Can you work these out from the model? Positions are in its coordinate system, mm. Coordinates: 2 decimals unless noted, no trailing zeros. Order: outer loops, then holes, each group sorted by start corner. A loop starts at its lowest first (then second) coordinate and runs counter-clockwise, first axis right, second up. Notation, with made-up numbers: (77.25, 86) -> (92.25, 86) arc R18 cw to (92.25, 112) -> close; hole circle Ø1 at (-32.75, 25.5). An arc over 180 degrees is marked (long way). Answer in a Markdown table with one row per item. Add a question column.
1. Imagine slicing it at B-B on x = 2.54. Write out the boundary of the cut face in (y, z), plus the area to 3 significant figures.
2. Will this pin go through, and if not, where does the flat tip stop? pin 1 (2.5 mm diameter, centred on x = 2.54, z = -3.048, fed in from +Y).
3. If I drill on line 1 along X through (y, z) = (0.45, -10.75); line 2 along X through (y, z) = (0.75, -12); line 3 along Z through (x, y) = (3.5, 0.25), over which ranges is the centre line in solid material (lowest first)? Write a range as [from, to].
4. Imagine slicing it at D-D on z = -6.25. Write out the boundary of the cut face in (x, y), plus the area to 3 significant figures.
5. We'd pull the mould along Z, two halves only. Please class faces 1 (the face through (13, 1, 0)), 2 (the face through (12.878, 1.252, -7.536)), 3 (the face through (2.998, 1.252, -9.214)): pulls with the +Z half, pulls with the -Z half, needs draft (parallel to the pull), parting line crosses it, or undercut.
6. Imagine slicing it at C-C on z = -11.75. Write out the boundary of the cut face in (x, y), plus the area to 3 significant figures.
7. Imagine slicing it at A-A on y = 2. Write out the boundary of the cut face in (x, z), plus the area to 3 significant figures.
from build123d import *

# Parameters (mm, degrees)
SKETCH1_R           = 1.524
BOSS_EXTRUDE1_DEPTH = 2.54


with BuildPart() as part:
    # Sketch1 → Boss-Extrude1 (new body)
    with BuildSketch(Plane(origin=(0, 0, 0), x_dir=(1, 0, 0), z_dir=(0, 1, 0))):
        Polygon((0, 0), (25.4, 0), (0, 15.285917978), align=None)
        with Locations(Location((2.54, 3.048, 0), (0, 0, 270))):
            Circle(SKETCH1_R, mode=Mode.SUBTRACT)
        with Locations(Location((2.54, 10.668, 0), (0, 0, 270))):
            Circle(SKETCH1_R, mode=Mode.SUBTRACT)
    extrude(amount=BOSS_EXTRUDE1_DEPTH)


solid = part.part
Answers follow:
| question | item | result |
|---|---|---|
| 1 | outline | (0, -13.76) -> (2.54, -13.76) -> (2.54, -12.19) -> (0, -12.19) -> close; (0, -9.14) -> (2.54, -9.14) -> (2.54, -4.57) -> (0, -4.57) -> close; (0, -1.52) -> (2.54, -1.52) -> (2.54, 0) -> (0, 0) -> close |
| 1 | area | 19.5 mm² |
| 2 | pin 1 | passes through |
| 3 | line 1 | x = [0, 1.02], [4.06, 7.54] |
| 3 | line 2 | x = [0, 1.8], [3.28, 5.46] |
| 3 | line 3 | z = [-13.18, -11.85], [-9.48, -4.23], [-1.86, 0] |
| 4 | outline | (0, 0) -> (15.01, 0) -> (15.01, 2.54) -> (0, 2.54) -> close |
| 4 | area | 38.1 mm² |
| 5 | face 1 | pulls with the +Z half |
| 5 | face 2 | pulls with the -Z half |
| 5 | face 3 | undercut |
| 6 | outline | (0, 0) -> (1.47, 0) -> (1.47, 2.54) -> (0, 2.54) -> close; (3.61, 0) -> (5.88, 0) -> (5.88, 2.54) -> (3.61, 2.54) -> close |
| 6 | area | 9.47 mm² |
| 7 | outline | (0, -15.29) -> (25.4, 0) -> (0, 0) -> close; hole circle Ø3.05 at (2.54, -10.67); hole circle Ø3.05 at (2.54, -3.05) |
| 7 | area | 180 mm² |
